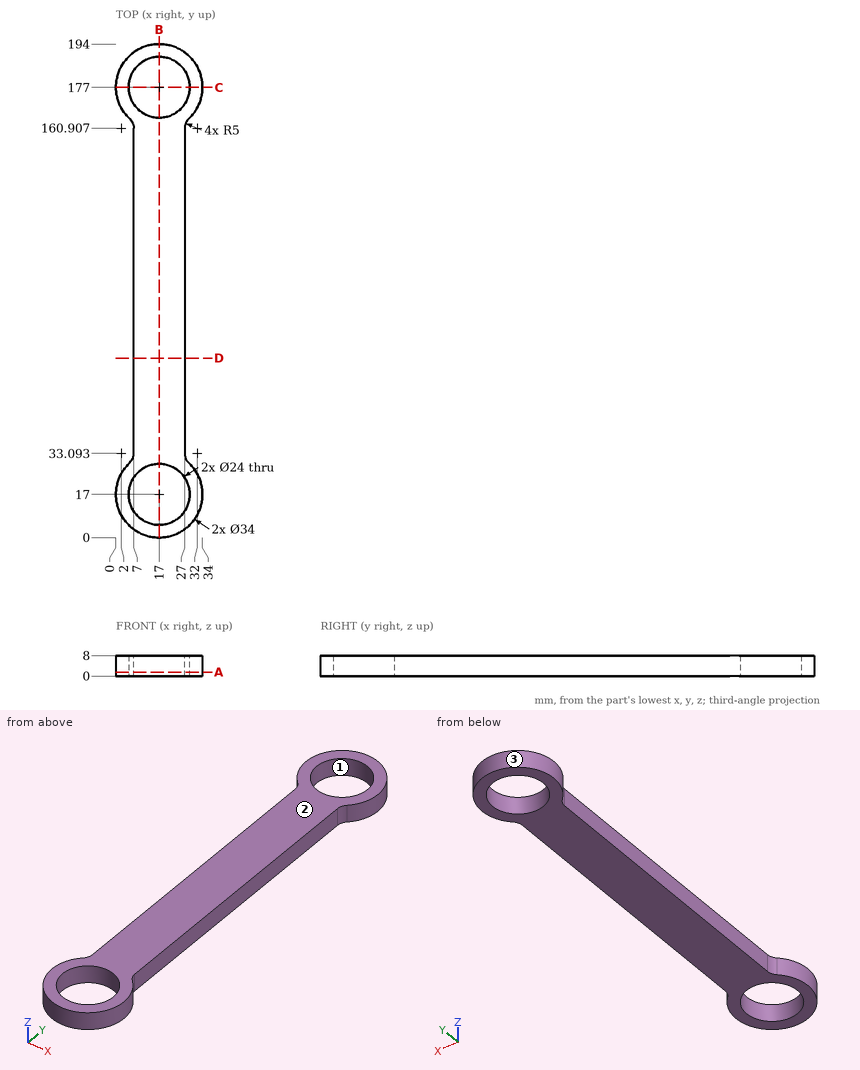
The drawing under review shows one solid part. Ordinate dimensions are in mm from its lowest x, y, z. Round coordinates to 2 decimals unless told otherwise and drop trailing zeros. Write each loop counter-clockwise with the first axis right and the second up, starting at its lowest first coordinate (ties: lowest second). Pieces come first, ordered by that corner, then holes. Notation, with made-up numbers: (-5, -16) - (36, -16) arc R23 cw to (36, 18) - close; hole circle Ø7 at (57.5, -35). An arc over 180 degrees is marked (long way). Use a Markdown table: item, result. Add a question column.
1. Clearance check with flat-ended pins moving along their axes: pin 1 (19 mm diameter, centred on x = 17, y = 177, fed in from +Z) (3 decimals); pin 2 (1 mm diameter, centred on x = 16.5, y = 66.5, fed in from -Z); pin 3 (2 mm diameter, centred on y = 82.5, z = 6.5, fed in from +X); pin 4 (4 mm diameter, centred on y = 114.5, z = 4, fed in from -X). State where each tip first meets the part, or that it passes through.
2. We need section D-D (y = 70.5). State the section outline as (x, z) points.
3. We need section C-C (y = 177). State the section outline as (x, z) points, then the cut area to 3 significant figures.
4. We need section B-B (x = 17). State the section outline as (y, z) points.
5. Mouldability with a two-part tool opening along X and no side actions: class the marked faces 1, 2 and 3 as +X half, -X half, draft (parallel to the pull), parting line (faces both ways), or undercut.
6. We need section A-A (z = 1.5). State the section outline as (x, y) points (1 decimal).
7. Wall thickness on probe 1 along Y at (x, z) = (17, 4.25); probe 2 along Y at (x, z) = (23.5, 4) (1 decimal); probe 3 along X at (y, z) = (17, 2.75): over which ranges is each line inside the solid? List them lowest first.
Output:
| question | item | result |
|---|---|---|
| 1 | pin 1 | passes through |
| 1 | pin 2 | stops at z = 0 |
| 1 | pin 3 | stops at x = 27 |
| 1 | pin 4 | stops at x = 7 |
| 2 | outline | (7, 0) - (27, 0) - (27, 8) - (7, 8) - close |
| 3 | outline | (0, 0) - (5, 0) - (5, 8) - (0, 8) - close; (29, 0) - (34, 0) - (34, 8) - (29, 8) - close |
| 3 | area | 80.0 mm2 |
| 4 | outline | (0, 0) - (5, 0) - (5, 8) - (0, 8) - close; (29, 0) - (165, 0) - (165, 8) - (29, 8) - close; (189, 0) - (194, 0) - (194, 8) - (189, 8) - close |
| 5 | face 1 | undercut |
| 5 | face 2 | draft |
| 5 | face 3 | parting line |
| 6 | outline | (5.4, 29.4) arc R17 ccw (long way) to (28.6, 29.4) arc R5 cw to (27, 33.1) - (27, 160.9) arc R5 cw to (28.6, 164.6) arc R17 ccw (long way) to (5.4, 164.6) arc R5 cw to (7, 160.9) - (7, 33.1) arc R5 cw to start; hole circle Ø24 at (17, 17); hole circle Ø24 at (17, 177) |
| 7 | probe 1 | y = 0 to 5, 29 to 165, 189 to 194 |
| 7 | probe 2 | y = 1.3 to 6.9, 27.1 to 166.9, 187.1 to 192.7 |
| 7 | probe 3 | x = 0 to 5, 29 to 34 |
